Design review of the part shown in the three views and the two pictorial views. Dimensions are in mm from the part's minimum x, y and z. A direction names the side the tool comes from. Coordinates: 2 decimals unless noted, no trailing zeros. Loops run counter-clockwise (first coordinate to the right, second up) from the corner with the lowest first, then second, coordinate; pieces in that order, holes last. Notation, with made-up numbers: M 60.25,43 L 89.25,43 A28 ccw 89.25,73 Z; hole C -1,12 d6. An arc over 180 degrees is marked long. Put each result on its own line as item: value. Start each with the question number.
(1) Take a section at D-D, the plane x = 37. Give the boundary of the cut face in (y, z).
(2) Take a section at B-B, the plane x = 60. Give the boundary of the cut face in (y, z), then the cut area to 3 significant figures.
(3) For the marked faces 1 and 2, list the 3-axis set-ups (+Z, -Z, +X, -X, +Y, -Y) from which the entire face can be reached by the end or side of a thin tool; tool diameter is ignored.
(4) For probe 1 along Y at (x, z) = (31, 108); probe 2 along X at (y, z) = (36, 119); probe 3 along Z at (x, y) = (63.5, 30), list the stretches that pass through material, from the lowest coordinate up. Write a range as [from, to].
(5) Clearance check with flat-ended pins moving along their axes: pin 1 (1.9 mm diameter, centred on y = 21.5, z = 79, fed in from -X); pin 2 (5.5 mm diameter, centred on x = 158, y = 30, fed in from +Z); pin 3 (13 mm diameter, centred on y = 15.5, z = 121.5, fed in from -X); pin 4 (2 mm diameter, centred on y = 44, z = 80, fed in from -X). State where each tip first meets the part, or that it passes through.
(6) Take a section at A-A, the plane y = 32. Give the boundary of the cut face in (x, z).
(7) Take a section at C-C, the plane z = 70. Give the boundary of the cut face in (x, y), then the cut area to 3 significant figures.
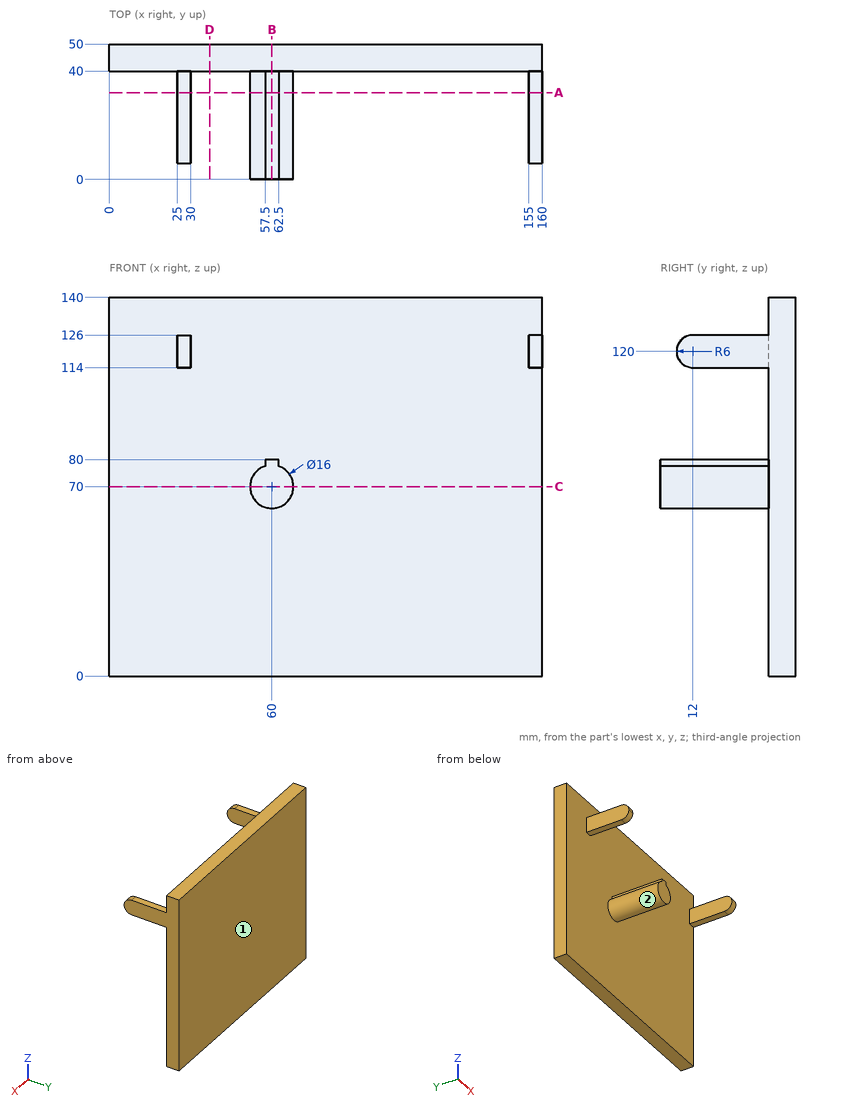
Computed values:
1. outline: M 40,0 L 50,0 L 50,140 L 40,140 Z
2. outline: M 0,62 L 40,62 L 40,0 L 50,0 L 50,140 L 40,140 L 40,80 L 0,80 Z
2. area: 2,120 mm^2
3. face 1: +Z, -Z, +X, -X, +Y
3. face 2: -Y
4. probe 1: y = [40, 50]
4. probe 2: x = [25, 30], [155, 160]
4. probe 3: z = [62.81, 77.19]
5. pin 1: stops at x = 57.5
5. pin 2: stops at z = 126
5. pin 3: stops at x = 25
5. pin 4: stops at x = 0
6. outline: M 25,114 L 30,114 L 30,126 L 25,126 Z; M 57.5,77.6 A8 ccw long 62.5,77.6 L 62.5,80 L 57.5,80 Z; M 155,114 L 160,114 L 160,126 L 155,126 Z
7. outline: M 0,40 L 52,40 L 52,0 L 68,0 L 68,40 L 160,40 L 160,50 L 0,50 Z
7. area: 2,240 mm^2
